from build123d import *

# Parameters (mm, degrees)
BOSS_EXTRUDE1_DEPTH = 25.4
SKETCH1_3_R         = 4.7625
CUT_EXTRUDE1_DEPTH  = 22.225
SKETCH2_R           = 6.0325
CUT_EXTRUDE2_DEPTH  = 4.175
SKETCH3_W           = 3.175
SKETCH3_H           = 22.225
CUT_EXTRUDE4_DEPTH  = 26.4
SKETCH4_R           = 6.35
CUT_EXTRUDE5_DEPTH  = 30.1752


with BuildPart() as part:
    # Sketch1 → Boss-Extrude1 (new body)
    with BuildSketch(Plane.XY):
        with BuildLine():
            Line((-12.7, 0), (12.7, 0))
            Line((12.7, 0), (12.7, 46.99))
            ThreePointArc((12.7, 46.99), (9.724204897, 54.174204897), (2.54, 57.15))
            Line((2.54, 57.15), (-2.54, 57.15))
            ThreePointArc((-2.54, 57.15), (-9.724204897, 54.174204897), (-12.7, 46.99))
            Line((-12.7, 46.99), (-12.7, 0))
        make_face()
    extrude(amount=-BOSS_EXTRUDE1_DEPTH)

    # Sketch1<3> → Cut-Extrude1 (cut)
    with BuildSketch(Plane.XY):
        with Locations((0, 41.275)):
            Circle(SKETCH1_3_R)
    extrude(amount=-CUT_EXTRUDE1_DEPTH, mode=Mode.SUBTRACT)

    # Sketch2 → Cut-Extrude2 (cut, through all)
    with BuildSketch(Plane.XY.offset(-22.225)):
        with Locations((0, 41.275)):
            Circle(SKETCH2_R)
    extrude(amount=-CUT_EXTRUDE2_DEPTH, mode=Mode.SUBTRACT)

    # Sketch3 → Cut-Extrude4 (cut, through all)
    with BuildSketch(Plane(origin=(12.7, 0, 0), x_dir=(0, 0, -1), z_dir=(1, 0, 0))):
        with Locations((1.5875, 11.1125)):
            Rectangle(SKETCH3_W, SKETCH3_H)
    extrude(amount=-CUT_EXTRUDE4_DEPTH, mode=Mode.SUBTRACT)

    # Sketch4 → Cut-Extrude5 (cut)
    with BuildSketch(Plane.XZ):
        with Locations((0, -12.7)):
            Circle(SKETCH4_R)
    extrude(amount=-CUT_EXTRUDE5_DEPTH, mode=Mode.SUBTRACT)


solid = part.part
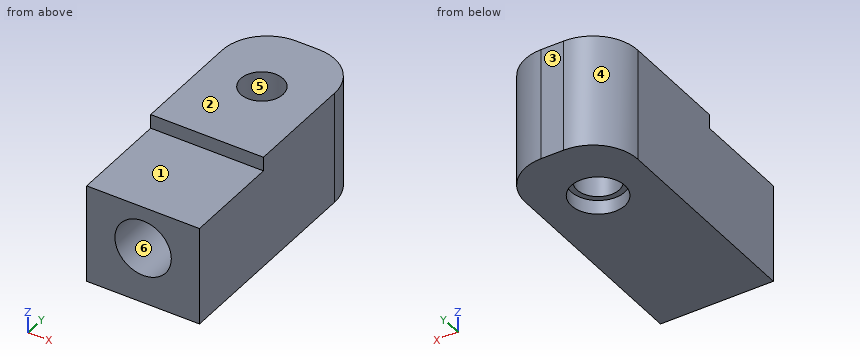
Geometry check sheet. Reference: the model listing, model coordinates, mm. Face numbers are marked on the shaded views. A direction names the side the tool comes from. Give positions to 0.01 mm unless a question says otherwise; leave off trailing zeros. Loops run counter-clockwise (first coordinate to the right, second up) from the corner with the lowest first, then second, coordinate; pieces in that order, holes last. Notation, with made-up numbers: M -20,-26 L 30,-26 A19 cw 30,-8 Z; hole C -24,70 d7. An arc over 180 degrees is marked long. Answer as a JSON object with one key per item and string values. Group by question number.
Item 1: Access from +Z, -Z, +X, -X, +Y, -Y to the whole of each face (thin tool, end or side, straight path). Record for the marked faces 1 and 2.
Item 2: Mould release check, pull along X, two halves, no side actions. Record for the marked faces 3, 4, 5 and 6: pulls with the +X half, pulls with the -X half, needs draft (parallel to the pull), parting line crosses it, or undercut.
Item 3: Gauge pin test, flat ends, axial feed: pin 1 (6.5 mm diameter, centred on x = 3, z = -13, fed in from -Y); pin 2 (10 mm diameter, centred on x = 8, y = 11.5, fed in from +Z) (3 decimals). Record the tip position at first contact, or that the pin passes through.
Item 4: Sectioned sample at C-C on y = 26. Record the boundary of the cut face in (x, z).
Item 5: Material ranges on L1, parallel to Y at x = 0, z = -7.25; L2, parallel to X at y = 5, z = -13; L3, parallel to Z at x = 0, y = 8 (3 decimals), recorded low to high.
Findings below:
{
 "1": {"face 1": "+Z, +X, -X, -Y", "face 2": "+Z, +X, -X, +Y, -Y"},
 "2": {"face 3": "needs draft", "face 4": "pulls with the -X half", "face 5": "undercut", "face 6": "undercut"},
 "3": {"pin 1": "y = 30.18", "pin 2": "z = -3.175"},
 "4": {"outline": "M -12.7,-25.4 L 12.7,-25.4 L 12.7,0 L -12.7,0 Z; hole C 0,-12.7 d12.7"},
 "5": {"L1": "30.18 to 36.51, 46.04 to 57.15", "L2": "-12.7 to -6.34, 6.34 to 12.7", "L3": "-25.4 to -19.05, -6.35 to -3.175"}
}
